```python
from build123d import *

# Parameters (mm, degrees)
F2_R   = 9.525
F2_R_2 = 8.525


with BuildPart() as f3:
    # F3: sweep along a path in F0
    with BuildLine(Plane.XZ) as f3_path:
        Line((120, 120), (59.525, 120))
        ThreePointArc((59.525, 120), (17.4344688499, 102.5655311501), (0, 60.475))
        Line((0, 60.475), (0, 0))
    # F2 (on plane+point) → F3 (sweep)
    with BuildSketch(Plane.YZ.offset(120)):
        with Locations((0, 120)):
            Circle(F2_R)
        with Locations((0, 120)):
            Circle(F2_R_2, mode=Mode.SUBTRACT)
    sweep(path=f3_path.line)


solid = f3.part
```
CAD build for the part. Positions are in the model's coordinates, mm. A direction names the side the tool comes from. Give positions to 0.01 mm unless a question says otherwise; leave off trailing zeros. Order: outer loops, then holes, each group sorted by start corner. A loop starts at its lowest first (then second) coordinate and runs counter-clockwise, first axis right, second up.
(1) Mould opens along Y. For faces 3 (the cylindrical face through (89.34, -1.85, 128.32)), 4 (the cylindrical face through (89.339, -1.24, 110.556)), 5 (the flat face through (-9, 1, 0)) say: released by +Y, released by -Y, zero draft, split by the parting line, or undercut.
(2) Drill centre lines: L1, parallel to X at y = 0, z = 43 (3 decimals); L2, parallel to Z at x = 107, y = 0 (3 decimals). Where is each one in solid material? Low to high.
(3) Saw through at B-B, the plane x = 65. Give the cut face in (y, z) (3 decimals), then the cut area to 3 significant figures.
(4) Saw through at A-A, the plane y = 0. Give the cut face in (x, z) (3 decimals), then the cut area to 3 significant figures.
(5) Tool access for faces 1 (the cylindrical face through (8.452, -1.11, 29.814)), 2 (the flat face through (120, -1, 111)): list every direction of +Z, -Z, +X, -X, +Y, -Y with a clear straight run to the whole face (end or side of a thin tool).
(6) Saw through at C-C, the plane z = 54. Give the cut face in (x, y) (3 decimals), then the cut area to 3 significant figures.
(7) Flat gauge pins, fed straight in: pin 1 (2 mm diameter, centred on y = -6.5, z = 74, fed in from +X); pin 2 (1.5 mm diameter, centred on x = 59.5, y = 1.5, fed in from +Z); pin 3 (1.5 mm diameter, centred on x = 32, y = 1.5, fed in from -Z). Where does each tip first touch, or does it go through?
Results found:
1. face 3: undercut
1. face 4: split by the parting line
1. face 5: zero draft
2. L1: x = -9.525 to -8.525, 8.525 to 9.525
2. L2: z = 110.475 to 111.475, 128.525 to 129.525
3. outline: circle Ø19.05 at (0, 120); hole circle Ø17.05 at (0, 120)
3. area: 56.7 mm2
4. outline: (-9.525, 0) - (-8.525, 0) - (-8.525, 60.475) arc R68.05 cw to (59.525, 128.525) - (120, 128.525) - (120, 129.525) - (59.525, 129.525) arc R69.05 ccw to (-9.525, 60.475) - close; (8.525, 0) - (9.525, 0) - (9.525, 60.475) arc R50 cw to (59.525, 110.475) - (120, 110.475) - (120, 111.475) - (59.525, 111.475) arc R51 ccw to (8.525, 60.475) - close
4. area: 429 mm2
5. face 1: -Z
5. face 2: +Z, -Z, +X, +Y, -Y
6. outline: circle Ø19.05 at (0, 0); hole circle Ø17.05 at (0, 0)
6. area: 56.7 mm2
7. pin 1: stops at x = 9.62
7. pin 2: stops at z = 129.5
7. pin 3: stops at z = 101.84
